Could you check a few things on this model? Use its own coordinates, in mm. A direction names the side the tool comes from. Coordinates: 2 decimals unless noted, no trailing zeros. Write each loop counter-clockwise with the first axis right and the second up, starting at its lowest first coordinate (ties: lowest second). Pieces come first, ordered by that corner, then holes. Notation, with made-up numbers: (45.25, 16.5) - (81.25, 16.5) arc R20 cw to (81.25, 26.5) - close; hole circle Ø11 at (-29.5, 9). An arc over 180 degrees is marked (long way). Answer as a JSON object with one key per item and string values. Group by question number.
1) We'd pull the mould along Z, two halves only. Please class faces 4 (the flat face through (-10, 72, -39)), 5 (the flat face through (-55.338, 44, 11)), 6 (the flat face through (-1, 44, 30)), 7 (the flat face through (-1, 40, -40)): released by +Z, released by -Z, zero draft, split by the parting line, or undercut.
2) If we section it at A-A (y = 8.5): Write out the boundary of the cut face in (x, z), plus the area to 3 significant figures.
3) Will these pins go through, and if not, where does the flat tip stop? pin 1 Ø2.5 at (x, y) = (30.9, 8.5) entering from -Z; pin 2 Ø5 at (x, z) = (51, -28.5) entering from +Y.
4) If we section it at D-D (z = -29.5): Write out the boundary of the cut face in (x, y).
5) Please list where these lines run through material, in increasing order: line 1 along Z through (x, y) = (-5, 47.5); line 2 along X through (y, z) = (76.5, -37.65); line 3 along Y through (x, z) = (30.9, -37.55).
6) If we section it at B-B (x = 30.9): Write out the boundary of the cut face in (y, z), plus the area to 4 significant figures.
7) On a 3-axis mill with a long thin cutter (end or side, diameter ignored), from which of +Z, -Z, +X, -X, +Y, -Y can I reach the whole of each face in a straight line? I mean faces 1 (the flat face through (35, 44, -13)), 2 (the flat face through (-1, 82, -9)), 3 (the flat face through (-51, 60, -39)). Say none if no direction works.
8) If we section it at C-C (x = 15.5): Write out the boundary of the cut face in (y, z), plus the area to 3 significant figures.
```python
from build123d import *

# Parameters (mm, degrees)
ESQUISSE1_W              = 130
ESQUISSE1_H              = 80
BOSS_EXTRU_1_DEPTH       = 82
ESQUISSE4_W              = 110
ESQUISSE4_H              = 19
ENL_V_MAT_EXTRU_1_DEPTH  = 77
ESQUISSE7_W              = 80
ESQUISSE7_H              = 24
ENL_V_MAT_EXTRU_2_DEPTH  = 5
ESQUISSE8_W              = 80
ESQUISSE8_H              = 24
ENL_V_MAT_EXTRU_3_DEPTH  = 5
CONG_1_R                 = 2
ESQUISSE9_W              = 110.509811946
ESQUISSE9_H              = 38
ENL_V_MAT_EXTRU_4_DEPTH  = 77
ESQUISSE10_W             = 20
ESQUISSE10_H             = 10
ENL_V_MAT_EXTRU_5_DEPTH  = 77
ESQUISSE11_R             = 1.5
ENL_V_MAT_EXTRU_6_DEPTH  = 3
ESQUISSE12_R             = 1.5
ENL_V_MAT_EXTRU_7_DEPTH  = 3
ESQUISSE13_R             = 1.5
ENL_V_MAT_EXTRU_8_DEPTH  = 3
ESQUISSE14_R             = 1.5
ENL_V_MAT_EXTRU_11_DEPTH = 3


with BuildPart() as part:
    # Esquisse1 → Boss.-Extru.1 (new body)
    with BuildSketch(Plane(origin=(0, 0, 0), x_dir=(1, 0, 0), z_dir=(0, 1, 0))):
        Rectangle(ESQUISSE1_W, ESQUISSE1_H)
    extrude(amount=BOSS_EXTRU_1_DEPTH)

    # Esquisse4 → Enlèv. mat.-Extru.1 (cut)
    with BuildSketch(Plane(origin=(0, 82, 0), x_dir=(1, 0, 0), z_dir=(0, 1, 0))):
        with Locations((0, 27.5)):
            Rectangle(ESQUISSE4_W, ESQUISSE4_H)
    extrude(amount=-ENL_V_MAT_EXTRU_1_DEPTH, mode=Mode.SUBTRACT)

    # Esquisse7 → Enlèv. mat.-Extru.2 (cut)
    with BuildSketch(Plane(origin=(0, 0, -40), x_dir=(-1, 0, 0), z_dir=(0, 0, -1))):
        with Locations((11, 23)):
            Rectangle(ESQUISSE7_W, ESQUISSE7_H)
    extrude(amount=-ENL_V_MAT_EXTRU_2_DEPTH, mode=Mode.SUBTRACT)

    # Esquisse8 → Enlèv. mat.-Extru.3 (cut)
    with BuildSketch(Plane(origin=(0, 0, -40), x_dir=(-1, 0, 0), z_dir=(0, 0, -1))):
        with Locations((11, 60)):
            Rectangle(ESQUISSE8_W, ESQUISSE8_H)
    extrude(amount=-ENL_V_MAT_EXTRU_3_DEPTH, mode=Mode.SUBTRACT)

    # Congé1
    cong_1_edges = [part.edges().sort_by_distance(p)[0] for p in [
        (-65, 41, -40),
        (65, 41, -40),
        (65, 41, 40),
        (-65, 41, 40),
    ]]
    fillet(cong_1_edges, radius=CONG_1_R)

    # Esquisse9 → Enlèv. mat.-Extru.4 (cut)
    with BuildSketch(Plane(origin=(0, 82, 0), x_dir=(1, 0, 0), z_dir=(0, 1, 0))):
        with Locations((-0.082965324, -11)):
            Rectangle(ESQUISSE9_W, ESQUISSE9_H)
    extrude(amount=-ENL_V_MAT_EXTRU_4_DEPTH, mode=Mode.SUBTRACT)

    # Esquisse10 → Enlèv. mat.-Extru.5 (cut)
    with BuildSketch(Plane(origin=(0, 82, 0), x_dir=(1, 0, 0), z_dir=(0, 1, 0))):
        with Locations((45, 13)):
            Rectangle(ESQUISSE10_W, ESQUISSE10_H)
    extrude(amount=-ENL_V_MAT_EXTRU_5_DEPTH, mode=Mode.SUBTRACT)

    # Esquisse11 → Enlèv. mat.-Extru.6 (cut)
    with BuildSketch(Plane(origin=(0, 0, -40), x_dir=(-1, 0, 0), z_dir=(0, 0, -1))):
        with Locations((-30.9, 39.5)):
            Circle(ESQUISSE11_R)
    enl_v_mat_extru_6 = extrude(amount=-ENL_V_MAT_EXTRU_6_DEPTH, mode=Mode.SUBTRACT)

    # Esquisse12 → Enlèv. mat.-Extru.7 (cut)
    with BuildSketch(Plane(origin=(0, 0, -40), x_dir=(-1, 0, 0), z_dir=(0, 0, -1))):
        with Locations((-30.9, 45.5)):
            Circle(ESQUISSE12_R)
    enl_v_mat_extru_7 = extrude(amount=-ENL_V_MAT_EXTRU_7_DEPTH, mode=Mode.SUBTRACT)

    # Symétrie1: Enlèv. mat.-Extru.6, Enlèv. mat.-Extru.7 across plane
    add(enl_v_mat_extru_6.mirror(Plane(origin=(-11, 0, 0), x_dir=(0, 0, 1), z_dir=(1, 0, 0))), mode=Mode.SUBTRACT)
    add(enl_v_mat_extru_7.mirror(Plane(origin=(-11, 0, 0), x_dir=(0, 0, 1), z_dir=(1, 0, 0))), mode=Mode.SUBTRACT)

    # Esquisse13 → Enlèv. mat.-Extru.8 (cut)
    with BuildSketch(Plane(origin=(0, 0, -40), x_dir=(-1, 0, 0), z_dir=(0, 0, -1))):
        with Locations((-30.9, 76.5)):
            Circle(ESQUISSE13_R)
    enl_v_mat_extru_8 = extrude(amount=-ENL_V_MAT_EXTRU_8_DEPTH, mode=Mode.SUBTRACT)

    # Symétrie2: Enlèv. mat.-Extru.8 across plane
    add(enl_v_mat_extru_8.mirror(Plane(origin=(-11, 0, 0), x_dir=(0, 0, 1), z_dir=(1, 0, 0))), mode=Mode.SUBTRACT)

    # Esquisse14 → Enlèv. mat.-Extru.11 (cut)
    with BuildSketch(Plane(origin=(0, 0, -40), x_dir=(-1, 0, 0), z_dir=(0, 0, -1))):
        with Locations((-30.9, 8.5)):
            Circle(ESQUISSE14_R)
    enl_v_mat_extru_11 = extrude(amount=-ENL_V_MAT_EXTRU_11_DEPTH, mode=Mode.SUBTRACT)

    # Symétrie3: Enlèv. mat.-Extru.11 across plane
    add(enl_v_mat_extru_11.mirror(Plane(origin=(-11, 0, 0), x_dir=(0, 0, 1), z_dir=(1, 0, 0))), mode=Mode.SUBTRACT)


solid = part.part
```
Here are the results:
{
 "1": {"face 4": "zero draft", "face 5": "undercut", "face 6": "undercut", "face 7": "released by -Z"},
 "2": {"outline": "(-65, -38) arc R2 ccw to (-63, -40) - (-54.4, -40) - (-54.4, -37) - (-55, -37) - (-55, -18) - (35, -18) - (35, -8) - (-55.34, -8) - (-55.34, 30) - (55.17, 30) - (55.17, -8) - (55, -8) - (55, -37) - (32.4, -37) - (32.4, -40) - (63, -40) arc R2 ccw to (65, -38) - (65, 38) arc R2 ccw to (63, 40) - (-63, 40) arc R2 ccw to (-65, 38) - close; (-51.4, -40) - (29.4, -40) - (29.4, -37) - (-51.4, -37) - close", "area": "3,890 mm²"},
 "3": {"pin 1": "stops at z = -18", "pin 2": "stops at y = 5"},
 "4": {"outline": "(-65, 0) - (65, 0) - (65, 82) - (55, 82) - (55, 5) - (-55, 5) - (-55, 82) - (-65, 82) - close"},
 "5": {"line 1": "z = -40 to -37, -18 to -8, 30 to 40", "line 2": "x = -65 to -54.4, -51.4 to 29.4, 32.4 to 65", "line 3": "y = 0 to 7, 10 to 38, 41 to 44, 47 to 75, 78 to 82"},
 "6": {"outline": "(0, -40) - (7, -40) - (7, -37) - (5, -37) - (5, -18) - (82, -18) - (82, -8) - (5, -8) - (5, 30) - (82, 30) - (82, 40) - (0, 40) - close; (10, -40) - (38, -40) - (38, -37) - (10, -37) - close; (41, -40) - (44, -40) - (44, -37) - (41, -37) - close; (47, -40) - (75, -40) - (75, -37) - (47, -37) - close; (78, -40) - (82, -40) - (82, -37) - (78, -37) - close", "area": "2,135 mm²"},
 "7": {"face 1": "+Y", "face 2": "+Z, -Z, +X, -X, +Y", "face 3": "-Z"},
 "8": {"outline": "(0, -40) - (11, -40) - (11, -37) - (5, -37) - (5, -18) - (82, -18) - (82, -8) - (5, -8) - (5, 30) - (82, 30) - (82, 40) - (0, 40) - close; (35, -40) - (48, -40) - (48, -37) - (35, -37) - close; (72, -40) - (82, -40) - (82, -37) - (72, -37) - close", "area": "2,030 mm²"}
}
